from build123d import *

# Parameters (mm, degrees)
EXTRUDE_1_DEPTH     = 22.5
SKETCH_2_R          = 4
SKETCH_2_R_2        = 1.5
CUT_EXTRUDE_1_DEPTH = 45.2
CHAMFER_1_SIZE      = 4
SKETCH_4_R          = 1.5
CUT_EXTRUDE_2_DEPTH = 19
SKETCH_6_W          = 26.1795091
SKETCH_6_H          = 41
CUT_EXTRUDE_3_DEPTH = 10
CHAMFER_2_SIZE      = 4
CHAMFER_4_SIZE      = 4
FILLET_2_R          = 0.6
CHAMFER_5_SIZE      = 4
FILLET_3_R          = 0.6


with BuildPart() as part:
    # Sketch 1 → Extrude 1 (new body, symmetric)
    with BuildSketch(Plane.XY):
        Polygon((0, 0), (0, 48), (1.5, 48), (1.5, 1.5), (18, 1.5), (18, 0), align=None)
    extrude(amount=EXTRUDE_1_DEPTH, both=True)

    # Sketch 2 → Cut-Extrude 1 (cut)
    with BuildSketch(Plane(origin=(0, 1.5, 0), x_dir=(1, 0, 0), z_dir=(0, 1, 0))):
        with Locations((9, 0)):
            Circle(SKETCH_2_R)
        with Locations((9, 18.5)):
            Circle(SKETCH_2_R_2)
        with Locations((9, -18.5)):
            Circle(SKETCH_2_R_2)
        with BuildLine():
            Line((7.5, 8.1), (7.5, 12))
            ThreePointArc((7.5, 12), (9, 13.5), (10.5, 12))
            Line((10.5, 12), (10.5, 8.1))
            ThreePointArc((10.5, 8.1), (9, 6.6), (7.5, 8.1))
        make_face()
        with BuildLine():
            Line((10.5, -12), (10.5, -8.1))
            ThreePointArc((10.5, -8.1), (9, -6.6), (7.5, -8.1))
            Line((7.5, -8.1), (7.5, -12))
            ThreePointArc((7.5, -12), (9, -13.5), (10.5, -12))
        make_face()
    extrude(amount=-CUT_EXTRUDE_1_DEPTH, mode=Mode.SUBTRACT)

    # Chamfer 1
    chamfer_1_edges = [part.edges().sort_by_distance(p)[0] for p in [
        (0.75, 48, 22.5),
        (0.75, 48, -22.5),
        (18, 0.75, 22.5),
        (18, 0.75, -22.5),
    ]]
    chamfer(chamfer_1_edges, length=CHAMFER_1_SIZE)

    # Sketch 4 → Cut-Extrude 2 (cut, through all)
    with BuildSketch(Plane.ZY):
        with Locations((0, 42.5)):
            Circle(SKETCH_4_R)
        with Locations((0, 5.5)):
            Circle(SKETCH_4_R)
    extrude(amount=-CUT_EXTRUDE_2_DEPTH, mode=Mode.SUBTRACT)

    # Sketch 6 → Cut-Extrude 3 (cut)
    with BuildSketch(Plane.ZY):
        Polygon((7, 72.5), (7, 42.5), (33.1795091, 42.5), (33.38840833, 42.5), (33.38840833, 72.5), align=None)
        with Locations((20.08975455, 22)):
            Rectangle(SKETCH_6_W, SKETCH_6_H)
        with Locations((-20.08975455, 22)):
            Rectangle(SKETCH_6_W, SKETCH_6_H)
        Polygon((-33.38840833, 42.5), (-33.1795091, 42.5), (-7, 42.5), (-7, 72.5), (-33.38840833, 72.5), align=None)
    extrude(amount=-CUT_EXTRUDE_3_DEPTH, mode=Mode.SUBTRACT)

    # Chamfer 2
    chamfer_2_edges = [part.edges().sort_by_distance(p)[0] for p in [
        (0.75, 48, -7),
        (0.75, 48, 7),
    ]]
    chamfer(chamfer_2_edges, length=CHAMFER_2_SIZE)

    # Chamfer 4
    chamfer_4_edges = [part.edges().sort_by_distance(p)[0] for p in [
        (0.75, 1.5, -7),
        (0.75, 1.5, 7),
    ]]
    chamfer(chamfer_4_edges, length=CHAMFER_4_SIZE)

    # Fillet 2
    fillet_2_edges = [part.edges().sort_by_distance(p)[0] for p in [
        (1.5, 1.5, 0),
        (0.75, 48, -3),
        (0.75, 48, 3),
        (0.75, 44, 7),
        (0.75, 44, -7),
        (0.75, 1.5, -11),
        (0.75, 1.5, 11),
        (0.75, 5.5, 7),
        (0.75, 5.5, -7),
        (14, 0.75, 22.5),
        (14, 0.75, -22.5),
        (18, 0.75, 18.5),
        (18, 0.75, -18.5),
    ]]
    fillet(fillet_2_edges, radius=FILLET_2_R)

    # Chamfer 5
    chamfer_5_edges = [part.edges().sort_by_distance(p)[0] for p in [
        (0, 0.75, -22.5),
        (0, 0.75, 22.5),
    ]]
    chamfer(chamfer_5_edges, length=CHAMFER_5_SIZE)

    # Fillet 3
    fillet_3_edges = [part.edges().sort_by_distance(p)[0] for p in [
        (4, 0.75, 22.5),
        (0, 0.75, -18.5),
        (0, 0.75, 18.5),
        (4, 0.75, -22.5),
    ]]
    fillet(fillet_3_edges, radius=FILLET_3_R)


solid = part.part
Here's how the part is built. I have some questions about the finished solid (model axes, mm). A direction names the side the tool comes from. Coordinates: 2 decimals unless noted, no trailing zeros. Write each loop counter-clockwise with the first axis right and the second up, starting at its lowest first coordinate (ties: lowest second). Pieces come first, ordered by that corner, then holes. Notation, with made-up numbers: (-2.5, 33) - (41.5, 33) arc R24 ccw to (41.5, 57) - close; hole circle Ø3 at (82.25, -28). An arc over 180 degrees is marked (long way). Use one line per item in the form item = value.
1) On a 3-axis mill with a long thin cutter (end or side, diameter ignored), from which of +Z, -Z, +X, -X, +Y, -Y can I reach the whole of each face in a straight line? I mean faces 4 (the flat face through (18, 1, 0)), 5 (the flat face through (1, 24, -7)), 6 (the flat face through (7.5, 1, 10)). Say none if no direction works.
Solved:
face_4 = +Z, -Z, +X, +Y, -Y
face_5 = -Z, +X, -X, +Y
face_6 = +Y, -Y
2) I need wall thicknesses on line 1 (Z direction, x = 9, y = 0.5); line 2 (Y direction, x = 1.15, z = 0); line 3 (Y direction, x = 16.75, z = -3.5). Which ranges of each line are inside material? Lowest first, please.
Solved:
line_1 = -22.5 to -20, -17 to -13.5, -6.6 to -4, 4 to 6.6, 13.5 to 17, 20 to 22.5
line_2 = 0 to 4, 7 to 41, 44 to 48
line_3 = 0 to 1.5
3) Suppose I cut it at C-C, the plane y = 45.5. Write out the boundary of the cut face in (x, z), plus the area to 3 significant figures.
Solved:
outline = (0, -5.5) - (1.5, -5.5) - (1.5, 5.5) - (0, 5.5) - close
area = 16.5 mm2
4) Suppose I cut it at A-A, the plane x = 9. Write out the boundary of the cut face in (y, z), plus the area to 3 significant figures.
Solved:
outline = (0, -22.5) - (1.5, -22.5) - (1.5, -20) - (0, -20) - close; (0, -17) - (1.5, -17) - (1.5, -13.5) - (0, -13.5) - close; (0, -6.6) - (1.5, -6.6) - (1.5, -4) - (0, -4) - close; (0, 4) - (1.5, 4) - (1.5, 6.6) - (0, 6.6) - close; (0, 13.5) - (1.5, 13.5) - (1.5, 17) - (0, 17) - close; (0, 20) - (1.5, 20) - (1.5, 22.5) - (0, 22.5) - close
area = 25.8 mm2
5) Suppose I cut it at B-B, the plane x = 11.5. Write out the boundary of the cut face in (y, z), plus the area to 3 significant figures.
Solved:
outline = (0, -22.5) - (1.5, -22.5) - (1.5, -3.12) - (0, -3.12) - close; (0, 3.12) - (1.5, 3.12) - (1.5, 22.5) - (0, 22.5) - close
area = 58.1 mm2
6) Thinking about a two-plate mould opening in Y: for faces 1 (the flat face through (1, 48, 0)), 2 (the cylindrical face through (1, 4, 0)), 3 (the flat face through (0, 22, -1)), which applies, released by +Y, released by -Y, zero draft, split by the parting line, or undercut?
Solved:
face_1 = released by +Y
face_2 = undercut
face_3 = zero draft
7) I'm going to push flat-ended pins straight in: P1, Ø10, axis at x = 15, z = -12, coming from the +Y side; P2, Ø3, axis at x = 2.5, z = -11.5, coming from the +Y side; P3, Ø5, axis at y = 18.5, z = 3.5, coming from the +X side. Where does each tip first touch, or does it pass through?
Solved:
P1 = 1.5
P2 = 2.12
P3 = 1.5
